Read the model definition and answer for the solid it produces. Units are mm, in the model's axes. A direction names the side the tool comes from. Round coordinates to 2 decimals unless told otherwise and drop trailing zeros. Write each loop counter-clockwise with the first axis right and the second up, starting at its lowest first coordinate (ties: lowest second). Pieces come first, ordered by that corner, then holes. Notation, with made-up numbers: (-8.75, -35) - (35.25, -35) arc R23 cw to (35.25, -3) - close; hole circle Ø1 at (49.5, 71). An arc over 180 degrees is marked (long way). Use one line per item in the form item = value. Start each with the question number.
1) The part is cut by section D-D, the plane x = -3.75. Give the vertices of the cut face in (y, z).
2) For faces 1 (the face through (-4.05, 11, 3)), 2 (the face through (-5.864, 6.503, 0.517)), 3 (the face through (0, 13, 1.02)), determine the directions among +Z, -Z, +X, -X, +Y, -Y from which every point of the face is accessible in a straight line to the end or side of a thin tool.
3) The part is cut by section A-A, the plane y = 8.89. Give the vertices of the cut face in (x, z).
4) The part is cut by section C-C, the plane x = 2.54. Give the vertices of the cut face in (y, z), plus the area to 3 significant figures.
5) The part is cut by section B-B, the plane y = -11.43. Give the vertices of the cut face in (x, z).
6) For a pull along Y with two mould halves and no side action, classify faces 4 (the face through (0, 0, 0)), 5 (the face through (6.284, 11.936, 0.517)) as released by +Y, released by -Y, zero draft, split by the parting line, or undercut.
7) Consider line 1 along Z through (x, y) = (7.25, -9.25); line 2 along Y through (x, z) = (-3.75, 0.85); line 3 along X through (y, z) = (12.75, 3.35). Determine where each line is inside the solid, lowest interval first. Write a range as from..to.
8) Each of these flat-tipped pins is pushed along its axis until it touches: pin 1 (1.6 mm diameter, centred on x = 6.35, y = -1.27, fed in from +Z); pin 2 (1.1 mm diameter, centred on y = 12, z = 3.5, fed in from +X). Where does it stop, or does it pass through?
Autodesk Inventor part; units mm, degrees
ref_plane "YZ Plane" through (0, 0, 0) normal (1, 0, 0) x (0, 1, 0)
ref_plane "XZ Plane" through (0, 0, 0) normal (0, 1, 0) x (-1, 0, 0)
ref_plane "XY Plane" through (0, 0, 0) normal (0, 0, 1) x (1, 0, 0)
sketch "スケッチ1" plane through (0, 0, 0) normal (0, 0, 1) x (1, 0, 0)
  line L0 (-7.62, -12.7) -> (7.62, -12.7)
  line L1 (7.62, -12.7) -> (7.62, 12.7)
  line L2 (7.62, 12.7) -> (-7.62, 12.7)
  line L3 (-7.62, 12.7) -> (-7.62, -12.7)
  line L4 (-7.62, -12.7) -> (7.62, 12.7) construction
  line L5 (7.62, -12.7) -> (-7.62, 12.7) construction
  point P0 (0, 0)
  dimension "d0" = 15.24
  dimension "d1" = 25.4
extrude "押し出し1" add sketch "スケッチ1" along normal blind 1.02
sketch "スケッチ2" plane through (0, 0, 1.02) normal (0, 0, 1) x (1, 0, 0)
  line L0 (-6.35, -11.43) -> (6.35, -11.43) construction
  line L1 (6.35, -11.43) -> (6.35, 11.43) construction
  line L2 (6.35, 11.43) -> (-6.35, 11.43) construction
  line L3 (-6.35, 11.43) -> (-6.35, -11.43) construction
  line L4 (-6.35, -11.43) -> (6.35, 11.43) construction
  line L5 (6.35, -11.43) -> (-6.35, 11.43) construction
  line L6 (7.62, 12.7) -> (-7.62, 12.7) construction
  circle A0 centre (-6.35, 11.43) radius 0.51
  circle A1 centre (-6.35, 8.89) radius 0.51
  circle A2 centre (-6.35, 6.35) radius 0.51
  circle A3 centre (-6.35, 3.81) radius 0.51
  circle A4 centre (-6.35, 1.27) radius 0.51
  circle A5 centre (-6.35, -1.27) radius 0.51
  circle A6 centre (-6.35, -3.81) radius 0.51
  circle A7 centre (-6.35, -6.35) radius 0.51
  circle A8 centre (-6.35, -8.89) radius 0.51
  circle A9 centre (-6.35, -11.43) radius 0.51
  circle A10 centre (6.35, 11.43) radius 0.51
  circle A11 centre (6.35, 8.89) radius 0.51
  circle A12 centre (6.35, 6.35) radius 0.51
  circle A13 centre (6.35, 3.81) radius 0.51
  circle A14 centre (6.35, 1.27) radius 0.51
  circle A15 centre (6.35, -1.27) radius 0.51
  circle A16 centre (6.35, -3.81) radius 0.51
  circle A17 centre (6.35, -6.35) radius 0.51
  circle A18 centre (6.35, -8.89) radius 0.51
  circle A19 centre (6.35, -11.43) radius 0.51
  line L7 (-2.54, -11.43) -> (2.54, -11.43) construction
  line L8 (2.54, -11.43) -> (2.54, -8.89) construction
  line L9 (2.54, -8.89) -> (-2.54, -8.89) construction
  line L10 (-2.54, -8.89) -> (-2.54, -11.43) construction
  circle A20 centre (-2.54, -8.89) radius 0.51
  circle A21 centre (-2.54, -11.43) radius 0.51
  circle A22 centre (0, -8.89) radius 0.51
  circle A23 centre (0, -11.43) radius 0.51
  circle A24 centre (2.54, -8.89) radius 0.51
  circle A25 centre (2.54, -11.43) radius 0.51
  point P0 (0, 0)
  dimension "d4" = 12.7
  dimension "d5" = 1.27
  dimension "d6" = 1.02
  dimension "d9" = 2.54
  dimension "d12" = 12.7
  dimension "d15" = 3.81
  dimension "d16" = 5.08
  dimension "d19" = 2.54
  dimension "d22" = 2.54
extrude "押し出し2" cut sketch "スケッチ2" against normal blind 1.02
sketch "スケッチ3" plane through (0, 0, 1.02) normal (0, 0, 1) x (1, 0, 0)
  line L0 (-4.05, 8.2) -> (4.05, 8.2)
  line L1 (4.05, 8.2) -> (4.05, 13.8)
  line L2 (4.05, 13.8) -> (-4.05, 13.8)
  line L3 (-4.05, 13.8) -> (-4.05, 8.2)
  line L4 (-7.62, -12.7) -> (7.62, -12.7)
  point P0 (0, 0)
  point P1 (0, 8.2)
  dimension "d27" = 26.5
  dimension "d28" = 8.1
  dimension "d29" = 5.6
extrude "押し出し3" add sketch "スケッチ3" along normal blind 3.8
properties part number "Pololu_A_Star_32U4_Micro"
Geometry results:
q1.outline = (-12.7, 0) - (12.7, 0) - (12.7, 1.02) - (13.8, 1.02) - (13.8, 4.82) - (8.2, 4.82) - (8.2, 1.02) - (-12.7, 1.02) - close
q2.face_1 = +Z, -X, +Y, -Y
q2.face_2 = +Z, -Z
q2.face_3 = -Z, +X, -X, +Y
q3.outline = (-7.62, 0) - (-6.86, 0) - (-6.86, 1.02) - (-7.62, 1.02) - close; (-5.84, 0) - (5.84, 0) - (5.84, 1.02) - (4.05, 1.02) - (4.05, 4.82) - (-4.05, 4.82) - (-4.05, 1.02) - (-5.84, 1.02) - close; (6.86, 0) - (7.62, 0) - (7.62, 1.02) - (6.86, 1.02) - close
q4.outline = (-12.7, 0) - (-11.94, 0) - (-11.94, 1.02) - (-12.7, 1.02) - close; (-10.92, 0) - (-9.4, 0) - (-9.4, 1.02) - (-10.92, 1.02) - close; (-8.38, 0) - (12.7, 0) - (12.7, 1.02) - (13.8, 1.02) - (13.8, 4.82) - (8.2, 4.82) - (8.2, 1.02) - (-8.38, 1.02) - close
q4.area = 45.1 mm2
q5.outline = (-7.62, 0) - (-6.86, 0) - (-6.86, 1.02) - (-7.62, 1.02) - close; (-5.84, 0) - (-3.05, 0) - (-3.05, 1.02) - (-5.84, 1.02) - close; (-2.03, 0) - (-0.51, 0) - (-0.51, 1.02) - (-2.03, 1.02) - close; (0.51, 0) - (2.03, 0) - (2.03, 1.02) - (0.51, 1.02) - close; (3.05, 0) - (5.84, 0) - (5.84, 1.02) - (3.05, 1.02) - close; (6.86, 0) - (7.62, 0) - (7.62, 1.02) - (6.86, 1.02) - close
q6.face_4 = zero draft
q6.face_5 = undercut
q7.line_1 = 0..1.02
q7.line_2 = -12.7..12.7
q7.line_3 = -4.05..4.05
q8.pin_1 = 1.02
q8.pin_2 = 4.05
